Check sheet for the modelled part. Datum: model origin and axes. Units: mm. A direction names the side the tool comes from. Round coordinates to 2 decimals unless told otherwise and drop trailing zeros. Loops run counter-clockwise (first coordinate to the right, second up) from the corner with the lowest first, then second, coordinate; pieces in that order, holes last. Notation, with made-up numbers: (71, 16) -> (99, 16) arc R16 ccw to (99, 42) -> close; hole circle Ø4 at (66.25, 41.5). An arc over 180 degrees is marked (long way). Return JSON: item names as keys, results as strings.
from build123d import *

# Parameters (mm, degrees)
F0_W      = 57.15
F0_H      = 44.45
F1_DEPTH  = 25.4
F2_W      = 44.45
F2_H      = 31.75
F3_DEPTH  = 25.4
F5_DEPTH  = 25.4
F6_R      = 6.35
F7_DEPTH  = 25.4
F9_DEPTH  = 25.4
F11_DEPTH = 25.4


with BuildPart() as f1:
    # F0 (on Front) → F1 (new body)
    with BuildSketch(Plane.XZ):
        with Locations((28.575, 22.225)):
            Rectangle(F0_W, F0_H)
    extrude(amount=-F1_DEPTH)

    # F2 (on Front) → F3 (cut)
    with BuildSketch(Plane.XZ):
        with Locations((34.925, 28.575)):
            Rectangle(F2_W, F2_H)
    extrude(amount=-F3_DEPTH, mode=Mode.SUBTRACT)

    # F4 (on Top) → F5 (cut)
    with BuildSketch(Plane.XY):
        with BuildLine():
            ThreePointArc((50.8, 25.4), (55.474032, 19.799516), (57.15, 12.7))
            Line((57.15, 12.7), (57.15, 25.4))
            Line((57.15, 25.4), (50.8, 25.4))
        make_face()
        with BuildLine():
            ThreePointArc((57.15, 12.7), (55.474032, 5.600484), (50.8, 0))
            Line((50.8, 0), (57.15, 0))
            Line((57.15, 0), (57.15, 12.7))
        make_face()
    extrude(amount=F5_DEPTH, mode=Mode.SUBTRACT)

    # F6 (on Top) → F7 (cut)
    with BuildSketch(Plane.XY):
        with Locations((25.4, 12.7)):
            Circle(F6_R)
        with Locations((44.45, 12.7)):
            Circle(F6_R)
    extrude(amount=F7_DEPTH, mode=Mode.SUBTRACT)

    # F8 (on Right) → F9 (cut)
    with BuildSketch(Plane.YZ):
        with BuildLine():
            Line((19.05, 44.45), (6.35, 44.45))
            Line((6.35, 44.45), (6.35, 31.75))
            ThreePointArc((6.35, 31.75), (12.7, 25.4), (19.05, 31.75))
            Line((19.05, 31.75), (19.05, 44.45))
        make_face()
    extrude(amount=F9_DEPTH, mode=Mode.SUBTRACT)

    # F10 (on Right) → F11 (cut)
    with BuildSketch(Plane.YZ):
        with BuildLine():
            ThreePointArc((0, 38.1), (5.600484, 42.774032), (12.7, 44.45))
            Line((12.7, 44.45), (0, 44.45))
            Line((0, 44.45), (0, 38.1))
        make_face()
        with BuildLine():
            ThreePointArc((12.7, 44.45), (19.799516, 42.774032), (25.4, 38.1))
            Line((25.4, 38.1), (25.4, 44.45))
            Line((25.4, 44.45), (12.7, 44.45))
        make_face()
    extrude(amount=F11_DEPTH, mode=Mode.SUBTRACT)


solid = f1.part
Q1. Section check A-A (x = 25.4). Record the boundary of the cut face in (y, z), then the cut area to 3 significant figures.
Results list:
{"outline": "(0, 0) -> (6.35, 0) -> (6.35, 12.7) -> (0, 12.7) -> close; (19.05, 0) -> (25.4, 0) -> (25.4, 12.7) -> (19.05, 12.7) -> close", "area": "161 mm^2"}
Q2. Section check B-B (y = 16.5). Record the boundary of the cut face in (x, z).
Results list:
{"outline": "(0, 0) -> (20.31, 0) -> (20.31, 12.7) -> (12.7, 12.7) -> (12.7, 26.66) -> (0, 26.66) -> close; (30.49, 0) -> (39.36, 0) -> (39.36, 12.7) -> (30.49, 12.7) -> close; (49.54, 0) -> (56.69, 0) -> (56.69, 12.7) -> (49.54, 12.7) -> close"}
Q3. Material ranges on line 1 (X direction, y = 12.7, z = 5.25); line 2 (Y direction, x = 25.4, z = 6.5); line 3 (Z direction, x = 41.5, y = 22.75), recorded low to high.
Results list:
{"line 1": "0 to 19.05, 31.75 to 38.1, 50.8 to 57.15", "line 2": "0 to 6.35, 19.05 to 25.4", "line 3": "0 to 12.7"}
Q4. Section check D-D (x = 8.5). Record the boundary of the cut face in (y, z) (3 decimals).
Results list:
{"outline": "(0, 0) -> (25.4, 0) -> (25.4, 38.1) arc R15.875 ccw to (19.05, 43.125) -> (19.05, 31.75) arc R6.35 cw to (6.35, 31.75) -> (6.35, 43.125) arc R15.875 ccw to (0, 38.1) -> close"}
Q5. Draft check along Y on faces 1 (the cylindrical face through (20.72, 16.99, 6.26)), 2 (the flat face through (0, 13, 16)), 3 (the flat face through (19, 0, 11)). Enter one of: released by +Y, released by -Y, zero draft, split by the parting line, or undercut.
Results list:
{"face 1": "undercut", "face 2": "zero draft", "face 3": "released by -Y"}
Q6. Go/stop test with flat-tipped pins: pin 1 (12 mm diameter, centred on x = 50.5, y = 8.5, fed in from +Z); pin 2 (10 mm diameter, centred on x = 44.45, y = 12.7, fed in from +Z); pin 3 (5 mm diameter, centred on x = 7.5, y = 10, fed in from +Z); pin 4 (12 mm diameter, centred on y = 21, z = 33, fed in from +X). Record where each tip stops, or that it passes through.
Results list:
{"pin 1": "z = 12.7", "pin 2": "through", "pin 3": "z = 28.11", "pin 4": "x = 12.7"}
Q7. Section check C-C (z = 10). Record the boundary of the cut face in (x, y) (3 decimals).
Results list:
{"outline": "(0, 0) -> (50.8, 0) arc R15.875 ccw to (57.15, 12.7) arc R15.875 ccw to (50.8, 25.4) -> (0, 25.4) -> close; hole circle Ø12.7 at (25.4, 12.7); hole circle Ø12.7 at (44.45, 12.7)"}
Q8. Tool access check on faces 4 (the cylindrical face through (6.261, 22.506, 41.06)), 5 (the flat face through (12.7, 13, 24)), 6 (the flat face through (6, 6.35, 38)). Record the directions out of +Z, -Z, +X, -X, +Y, -Y that give a thin tool (end or side, any length) a straight path to the whole face; none if there is none.
Results list:
{"face 4": "+Z, +X, -X, +Y", "face 5": "+Z, +X, +Y, -Y", "face 6": "+Z, +X, -X"}
